Verification items for the finished model (mm, model axes). Face numbers are marked on the shaded views. Coordinates: 2 decimals unless noted, no trailing zeros. Write each loop counter-clockwise with the first axis right and the second up, starting at its lowest first coordinate (ties: lowest second). Pieces come first, ordered by that corner, then holes. Notation, with made-up numbers: M 8,47 L 35,47 A7 cw 35,55 Z; hole C 34.25,-23.75 d7. An arc over 180 degrees is marked long. One line per item, written item: value.
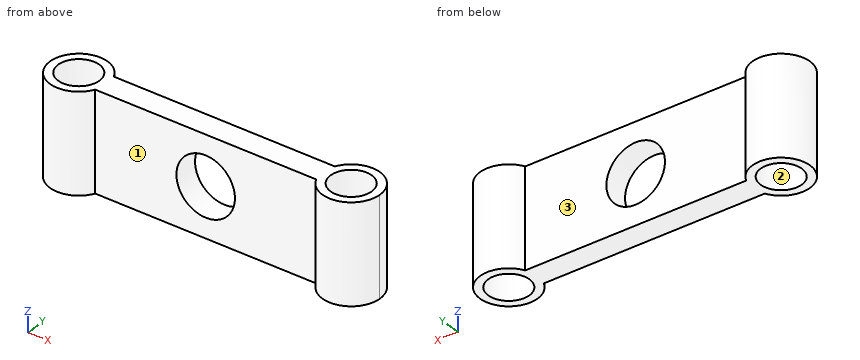
```python
from build123d import *

# Parameters (mm, degrees)
F1_DEPTH = 12
F2_D     = 5
F2_DEPTH = 15
F2_TIP   = 1.5021515476
F3_D     = 5
F3_DEPTH = 15
F3_TIP   = 1.5021515476
F5_D     = 7.2
F5_DEPTH = 10
F5_TIP   = 2.1630982285


# Not quite as in the source:
# - a feature names something its author has since deleted; it is built from what else it names


with BuildPart() as f1:
    # F0 (on Top) → F1 (new body)
    with BuildSketch(Plane.XY):
        with BuildLine():
            Line((-14.5, -1.8754155822), (-14.5, 1.1245844178))
            Line((-14.5, 1.1245844178), (-11.3377223398, 1.1245844178))
            ThreePointArc((-11.3377223398, 1.1245844178), (-18, -0.3754155822), (-11.3377223398, -1.8754155822))
            Line((-11.3377223398, -1.8754155822), (-14.5, -1.8754155822))
        make_face()
        with BuildLine():
            Line((-11.3377223398, 1.1245844178), (-14.5, 1.1245844178))
            Line((-14.5, 1.1245844178), (-14.5, -1.8754155822))
            Line((-14.5, -1.8754155822), (-11.3377223398, -1.8754155822))
            ThreePointArc((-11.3377223398, -1.8754155822), (-11.0854742781, -1.144189993), (-11, -0.3754155822))
            ThreePointArc((-11, -0.3754155822), (-11.0854742781, 0.3933588286), (-11.3377223398, 1.1245844178))
        make_face()
        with BuildLine():
            Line((15.8377223398, 1.1245844178), (-11.3377223398, 1.1245844178))
            ThreePointArc((-11.3377223398, 1.1245844178), (-11.0854742781, 0.3933588286), (-11, -0.3754155822))
            ThreePointArc((-11, -0.3754155822), (-11.0854742781, -1.144189993), (-11.3377223398, -1.8754155822))
            Line((-11.3377223398, -1.8754155822), (15.8377223398, -1.8754155822))
            ThreePointArc((15.8377223398, -1.8754155822), (15.5, -0.3754155822), (15.8377223398, 1.1245844178))
        make_face()
        with BuildLine():
            ThreePointArc((22.5, -0.3754155822), (19.7687744108, 3.0391101397), (15.8377223398, 1.1245844178))
            Line((15.8377223398, 1.1245844178), (19, 1.1245844178))
            Line((19, 1.1245844178), (19, -1.8754155822))
            Line((19, -1.8754155822), (15.8377223398, -1.8754155822))
            ThreePointArc((15.8377223398, -1.8754155822), (19.7687744108, -3.7899413041), (22.5, -0.3754155822))
        make_face()
        with BuildLine():
            Line((19, 1.1245844178), (15.8377223398, 1.1245844178))
            ThreePointArc((15.8377223398, 1.1245844178), (15.5, -0.3754155822), (15.8377223398, -1.8754155822))
            Line((15.8377223398, -1.8754155822), (19, -1.8754155822))
            Line((19, -1.8754155822), (19, 1.1245844178))
        make_face()
    extrude(amount=F1_DEPTH)

    # F2
    with Locations(Plane(origin=(0, 0, 0), x_dir=(1, 0, 0), z_dir=(0, 0, -1))):
        with Locations((19, 0.3754155822)):
            Hole(F2_D / 2, depth=F2_DEPTH)
            with Locations((0, 0, -(F2_DEPTH + F2_TIP / 2))):  # 118° drill point
                Cone(0, F2_D / 2, F2_TIP, mode=Mode.SUBTRACT)

    # F3
    with Locations(Plane(origin=(0, 0, 0), x_dir=(1, 0, 0), z_dir=(0, 0, -1))):
        with Locations((-14.5, 0.3754155822)):
            Hole(F3_D / 2, depth=F3_DEPTH)
            with Locations((0, 0, -(F3_DEPTH + F3_TIP / 2))):  # 118° drill point
                Cone(0, F3_D / 2, F3_TIP, mode=Mode.SUBTRACT)

    # F5
    with Locations(Plane(origin=(0, 1.1245844178, 0), x_dir=(-1, 0, 0), z_dir=(0, 1, 0))):
        with Locations((-2.25, 6)):
            Hole(F5_D / 2, depth=F5_DEPTH)
            with Locations((0, 0, -(F5_DEPTH + F5_TIP / 2))):  # 118° drill point
                Cone(0, F5_D / 2, F5_TIP, mode=Mode.SUBTRACT)


solid = f1.part
```
Item 1: Cross-section at C-C, the plane y = -1. Enter the section's corners in (x, z), and give its area (3 significant figures).
The answers:
outline: M -17.94,0 L -16.92,0 L -16.92,12 L -17.94,12 Z; M -12.08,0 L 16.58,0 L 16.58,12 L -12.08,12 Z; M 21.42,0 L 22.44,0 L 22.44,12 L 21.42,12 Z; hole C 2.25,6 d7.2
area: 328 mm²
Item 2: Cross-section at B-B, the plane z = 6. Enter the section's corners in (x, y).
The answers:
outline: M -11.34,-1.88 L -1.35,-1.88 L -1.35,1.12 L -11.34,1.12 A3.5 ccw long Z; M 5.85,-1.88 L 15.84,-1.88 A3.5 ccw long 15.84,1.12 L 5.85,1.12 Z; hole C -14.5,-0.38 d5; hole C 19,-0.38 d5
Item 3: Go/stop test with flat-tipped pins: P1, Ø3.5, axis at x = 6, z = 3, coming from the -Y side; P2, Ø3.5, axis at x = 7.5, z = 6, coming from the +Y side; P3, Ø2, axis at y = -3, z = 8.5, coming from the -X side. Record where each tip stops, or that it passes through.
The answers:
P1: stops at y = -1.88
P2: stops at y = 1.12
P3: stops at x = -17.6
Item 4: Scan lines: line 1 (X direction, y = -0.25, z = 11.75); line 2 (X direction, y = -1, z = 0.5); line 3 (Y direction, x = 19, z = 5.5). Record each from-to range of solid material in increasing order.
The answers:
line 1: x = -18 to -17, -12 to 16.5, 21.5 to 22.5
line 2: x = -17.94 to -16.92, -12.08 to 16.58, 21.42 to 22.44
line 3: y = -3.88 to -2.88, 2.12 to 3.12
Item 5: Cross-section at D-D, the plane z = 8.75. Enter the section's corners in (x, y).
The answers:
outline: M -11.34,-1.88 L -0.07,-1.88 L -0.07,1.12 L -11.34,1.12 A3.5 ccw long Z; M 4.57,-1.88 L 15.84,-1.88 A3.5 ccw long 15.84,1.12 L 4.57,1.12 Z; hole C -14.5,-0.38 d5; hole C 19,-0.38 d5
Item 6: Cross-section at A-A, the plane x = 2.25. Enter the section's corners in (y, z).
The answers:
outline: M -1.88,0 L 1.12,0 L 1.12,2.4 L -1.88,2.4 Z; M -1.88,9.6 L 1.12,9.6 L 1.12,12 L -1.88,12 Z
Item 7: Draft check along Y on the marked faces 1, 2 and 3. Enter one of: released by +Y, released by -Y, zero draft, split by the parting line, or undercut.
The answers:
face 1: released by -Y
face 2: undercut
face 3: released by +Y
